from build123d import *

# Parameters (mm, degrees)
SKETCH1_W           = 30
SKETCH1_H           = 70
BOSS_EXTRUDE1_DEPTH = 1
SKETCH2_W           = 30
SKETCH2_H           = 2.5
BOSS_EXTRUDE2_DEPTH = 1
SKETCH3_R           = 0.5
CUT_EXTRUDE1_DEPTH  = 30
SKETCH4_W           = 2.5
SKETCH4_H           = 2
CUT_EXTRUDE2_DEPTH  = 2.5
FILLET1_R           = 1
SKETCH5_W           = 30
SKETCH5_H           = 1
BOSS_EXTRUDE3_DEPTH = 5
FILLET2_R           = 1
SKETCH6_W           = 5
SKETCH6_H           = 2.5
CUT_EXTRUDE3_DEPTH  = 1
SKETCH7_W           = 30
SKETCH7_H           = 74.158210877
CUT_EXTRUDE4_DEPTH  = 0.2


with BuildPart() as part:
    # Sketch1 → Boss-Extrude1 (new body)
    with BuildSketch(Plane(origin=(0, 0, 0), x_dir=(1, 0, 0), z_dir=(0, 1, 0))):
        Rectangle(SKETCH1_W, SKETCH1_H)
    extrude(amount=BOSS_EXTRUDE1_DEPTH)

    # Sketch2 → Boss-Extrude2 (add)
    with BuildSketch(Plane(origin=(0, 1, 0), x_dir=(1, 0, 0), z_dir=(0, 1, 0))):
        with Locations((0, 33.75)):
            Rectangle(SKETCH2_W, SKETCH2_H)
    extrude(amount=BOSS_EXTRUDE2_DEPTH)

    # Sketch3 → Cut-Extrude1 (cut)
    with BuildSketch(Plane(origin=(15, 0, 0), x_dir=(0, 0, -1), z_dir=(1, 0, 0))):
        with Locations((33.75, 1)):
            Circle(SKETCH3_R)
    extrude(amount=-CUT_EXTRUDE1_DEPTH, mode=Mode.SUBTRACT)

    # Sketch4 → Cut-Extrude2 (cut)
    with BuildSketch(Plane(origin=(0, 0, -35), x_dir=(-1, 0, 0), z_dir=(0, 0, -1))):
        with Locations((-13.75, 1)):
            Rectangle(SKETCH4_W, SKETCH4_H)
        with Locations((13.75, 1)):
            Rectangle(SKETCH4_W, SKETCH4_H)
    extrude(amount=-CUT_EXTRUDE2_DEPTH, mode=Mode.SUBTRACT)

    # Fillet1
    fillet1_edges = [part.edges().sort_by_distance(p)[0] for p in [
        (0, 2, -35),
    ]]
    fillet(fillet1_edges, radius=FILLET1_R)

    # Sketch5 → Boss-Extrude3 (add)
    with BuildSketch(Plane.XY.offset(35)):
        with Locations((0, 0.5)):
            Rectangle(SKETCH5_W, SKETCH5_H)
    extrude(amount=BOSS_EXTRUDE3_DEPTH)

    # Fillet2
    fillet2_edges = [part.edges().sort_by_distance(p)[0] for p in [
        (0, 0, -35),
    ]]
    fillet(fillet2_edges, radius=FILLET2_R - 0.0001)  # a hair under: the kernel refuses the full size

    # Sketch6 → Cut-Extrude3 (cut)
    with BuildSketch(Plane(origin=(0, 1, 0), x_dir=(1, 0, 0), z_dir=(0, 1, 0))):
        with Locations((11.5, -37.75)):
            Rectangle(SKETCH6_W, SKETCH6_H)
    extrude(amount=-CUT_EXTRUDE3_DEPTH, mode=Mode.SUBTRACT)

    # Sketch7 → Cut-Extrude4 (cut)
    with BuildSketch(Plane.XZ):
        with Locations((0, 2.920894561)):
            Rectangle(SKETCH7_W, SKETCH7_H)
    extrude(amount=-CUT_EXTRUDE4_DEPTH, mode=Mode.SUBTRACT)


solid = part.part
Model file for the job. Use its own axes, mm. A direction names the side the tool comes from. Coordinates: 2 decimals unless noted, no trailing zeros. Order: outer loops, then holes, each group sorted by start corner. A loop starts at its lowest first (then second) coordinate and runs counter-clockwise, first axis right, second up. Notation, with made-up numbers: (-34, 15) -> (22, 15) arc R25 cw to (22, 53) -> close; hole circle Ø8 at (-23, 35). An arc over 180 degrees is marked (long way). Return JSON: item names as keys, results as strings. Group by question number.
Item 1: Wall check: line 1 along Y through (x, z) = (-3.5, -33.75); line 2 along Z through (x, y) = (13.5, 0.95); line 3 along Y through (x, z) = (2.25, 13.5). Give the ranges that are in metal, low to high. Write a range as [from, to].
Item 2: Flat gauge pins, fed straight in: P1, Ø0.9, axis at x = 14.5, y = 1, coming from the -Z side; P2, Ø10, axis at x = -7, z = -22.5, coming from the -Y side; P3, Ø5, axis at x = 1.5, z = 30.5, coming from the +Y side. Where does each tip first touch, or does it go through?
Item 3: Saw through at A-A on x = 11.5. State how many separate pieces and enclosed holes the cut face has, then the cut area to 3 significant figures.
Item 4: Tool access for faces 1 (the flat face through (0, 2, -33)), 2 (the flat face through (0, 0.2, 3)), 3 (the flat face through (0, 1, 3)), 4 (the flat face through (-12.5, 1, -33)), 5 (the flat face through (12.5, 1, -33)): list every direction of +Z, -Z, +X, -X, +Y, -Y with a clear straight run to the whole face (end or side of a thin tool).
Item 5: Saw through at C-C on z = -11. Write the cut outline in (x, y).
Values found:
{
 "1": {"line 1": "y = [0.2, 0.5], [1.5, 2]", "line 2": "z = [-32.5, 36.5], [39, 40]", "line 3": "y = [0.2, 1]"},
 "2": {"P1": "stops at z = -32.5", "P2": "stops at y = 0.2", "P3": "stops at y = 1"},
 "3": {"separate pieces": "2", "enclosed holes": "1", "area": "59.5 mm2"},
 "4": {"face 1": "+Z, -Z, +X, -X, +Y", "face 2": "+Z, +X, -X, -Y", "face 3": "+Z, +X, -X, +Y", "face 4": "-Z, -X, +Y, -Y", "face 5": "-Z, +X, +Y, -Y"},
 "5": {"outline": "(-15, 0.2) -> (15, 0.2) -> (15, 1) -> (-15, 1) -> close"}
}
